from build123d import *

# Parameters (mm, degrees)
BASE_FLANGE1_DEPTH = 741.4
EDGE_FLANGE1_DEPTH = 741.4
CUT_EXTRUDE3_DEPTH = 1


# Sheet-metal steps are written as plain solids
with BuildPart() as part:
    # Sketch1 → Base-Flange1 (new body)
    with BuildSketch(Plane.XY):
        with BuildLine():
            Line((-336.88, 0), (336.465786438, 0))
            ThreePointArc((336.465786438, 0), (336.84846987, -0.076120467), (337.172893219, -0.292893219))
            Line((337.172893219, -0.292893219), (407.700101013, -70.820101013))
            ThreePointArc((407.700101013, -70.820101013), (407.916873764, -71.144524361), (407.992994231, -71.527207794))
            Line((407.992994231, -71.527207794), (407.992994231, -102.112994231))
            Line((407.992994231, -102.112994231), (408.892994231, -102.112994231))
            Line((408.892994231, -102.112994231), (408.892994231, -71.527207794))
            ThreePointArc((408.892994231, -71.527207794), (408.748365343, -70.800109272), (408.336497116, -70.183704909))
            Line((408.336497116, -70.18370491), (337.809289322, 0.343502884))
            ThreePointArc((337.809289322, 0.343502884), (337.192884959, 0.755371112), (336.465786438, 0.9))
            Line((336.465786438, 0.9), (-336.88, 0.9))
            Line((-336.88, 0.9), (-336.88, 0))
        make_face()
    extrude(amount=BASE_FLANGE1_DEPTH)

    # Edge-Flange1 section (across the edge) → Edge-Flange1 (add)
    with BuildSketch(Plane(origin=(-337.88, 0, 741.4), x_dir=(1, 0, 0), z_dir=(0, 0, -1))):
        with BuildLine():
            Line((-0.9, 1), (-0.9, 31.6))
            Line((-0.9, 31.6), (0, 31.6))
            Line((0, 31.6), (0, 1))
            ThreePointArc((0, 1), (0.292893219, 0.292893219), (1, 0))
            Line((1, 0), (1, -0.9))
            ThreePointArc((1, -0.9), (-0.343502884, -0.343502884), (-0.9, 1))
        make_face()
    extrude(amount=EDGE_FLANGE1_DEPTH)

    # Sketch14 → Cut-Extrude3 (cut)
    with BuildSketch(Plane.XZ):
        Polygon((159.117677791, 526.822723002), (248.060263169, 717.560712871), (12.12, 717.560712871), (12.12, 25), (248.060263169, 25), (159.117677791, 215.737989869), align=None)
    extrude(amount=-CUT_EXTRUDE3_DEPTH, mode=Mode.SUBTRACT)


solid = part.part
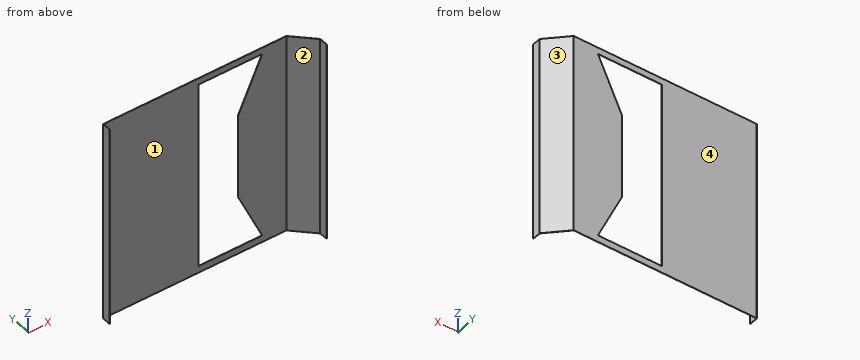
Design review of the part built by this model. Coordinates are the model's own, in mm. Face numbers are marked on the shaded views. Coordinates: 2 decimals unless noted, no trailing zeros. Order: outer loops, then holes, each group sorted by start corner. A loop starts at its lowest first (then second) coordinate and runs counter-clockwise, first axis right, second up.
Item 1: Take a section at C-C, the plane z = 682. Write out the cut boundary in (x, y), then the cut area to 3 significant figures.
Item 2: The part is to be moulded in two halves that separate along X. For the marked faces 1, 2, 3 and 4, say which applies: pulls with the +X half, pulls with the -X half, needs draft (parallel to the pull), parting line crosses it, or undercut.
Item 3: For line 1 (Y direction, x = 284, z = 622); line 2 (X direction, y = -21.5, z = 557.5); line 3 (X direction, y = -89.5, z = 79), list the stretches that pass through material, from the lowest coordinate up.
Item 4: Take a section at D-D, the plane y = -82. Write out the cut boundary in (x, z), then the cut area to 3 significant figures.
Item 5: For pin 1 Ø9 at (y, z) = (-22, 196) entering from +X; pin 2 Ø0.7 at (y, z) = (0.5, 462.5) entering from +X; pin 3 Ø0.7 at (y, z) = (0.5, 413) entering from -X, all flat-tipped, find the tip position at first contact; note any pin that passes through.
Item 6: Take a section at A-A, the plane z = 345.5. Write out the cut boundary in (x, y).
Item 7: Take a section at B-B, the plane x = 189. Write out the cut boundary in (y, z).
The answers:
1. outline: (-338.78, -31.6) - (-337.88, -31.6) - (-337.88, -1) arc R1 cw to (-336.88, 0) - (12.12, 0) - (12.12, 0.9) - (-336.88, 0.9) arc R1.9 ccw to (-338.78, -1) - close; (231.48, 0) - (336.47, 0) arc R1 cw to (337.17, -0.29) - (407.7, -70.82) arc R1 cw to (407.99, -71.53) - (407.99, -102.11) - (408.89, -102.11) - (408.89, -71.53) arc R1.9 ccw to (408.34, -70.18) - (337.81, 0.34) arc R1.9 ccw to (336.47, 0.9) - (231.48, 0.9) - close
1. area: 558 mm2
2. face 1: undercut
2. face 2: undercut
2. face 3: pulls with the +X half
2. face 4: needs draft
3. line 1: y = 0 to 0.9
3. line 2: x = -338.78 to -337.88, 358.38 to 359.65
3. line 3: x = 407.99 to 408.89
4. outline: (407.99, 0) - (408.89, 0) - (408.89, 741.4) - (407.99, 741.4) - close
4. area: 667 mm2
5. pin 1: stops at x = 364.65
5. pin 2: stops at x = 338
5. pin 3: stops at x = -338.39
6. outline: (-338.78, -31.6) - (-337.88, -31.6) - (-337.88, -1) arc R1 cw to (-336.88, 0) - (12.12, 0) - (12.12, 0.9) - (-336.88, 0.9) arc R1.9 ccw to (-338.78, -1) - close; (159.12, 0) - (336.47, 0) arc R1 cw to (337.17, -0.29) - (407.7, -70.82) arc R1 cw to (407.99, -71.53) - (407.99, -102.11) - (408.89, -102.11) - (408.89, -71.53) arc R1.9 ccw to (408.34, -70.18) - (337.81, 0.34) arc R1.9 ccw to (336.47, 0.9) - (159.12, 0.9) - close
7. outline: (0, 0) - (0.9, 0) - (0.9, 25) - (0, 25) - close; (0, 151.66) - (0.9, 151.66) - (0.9, 590.91) - (0, 590.91) - close; (0, 717.56) - (0.9, 717.56) - (0.9, 741.4) - (0, 741.4) - close
